Geometry: final body of the model. Coordinates: model frame, mm. Coordinates: 2 decimals unless noted, no trailing zeros. Order: outer loops, then holes, each group sorted by start corner. A loop starts at its lowest first (then second) coordinate and runs counter-clockwise, first axis right, second up. Notation, with made-up numbers: M 38.5,-34.5 L 46.5,-34.5 A24 ccw 46.5,-14.5 Z; hole C -19.75,-20.75 d7. An arc over 180 degrees is marked long. Use CSV: the item, a comma, the result in double quotes. Start each with the question number.
1. Section query B-B on z = 0.8. Return the cut outline in (x, y), and give its area (3 significant figures).
2. Section query D-D on x = -1200. Return the cut outline in (y, z), and give its area (3 significant figures).
3. Material intervals for line 1 (X direction, y = -220.5, z = 4.2); line 2 (Y direction, x = -1216.6, z = 3); line 3 (X direction, y = -244.5, z = 2.9), sorted ascending.
4. Section query C-C on x = -1019. Return the cut outline in (y, z), and give its area (3 significant figures).
5. Section query A-A on y = -232.5. Return the cut outline in (x, z), and give its area (4 significant figures).
6. First-contact query: P1, Ø4.5, axis at x = -957.6, y = -244.5, coming from the -Z side; P2, Ø1.5, axis at x = -1160, z = 1.5, coming from the +Y side. Flat tips, straight axial feed; report the tip coordinate or a pass-through.
from build123d import *

# Parameters (mm, degrees)
SKETCH1_W           = 267
SKETCH1_H           = 267.4
SKETCH1_R           = 2.5
SKETCH1_W_2         = 33
SKETCH1_H_2         = 90
BOSS_EXTRUDE1_DEPTH = 5
SKETCH6_W           = 267
SKETCH6_H           = 70.024397165
CUT_EXTRUDE4_DEPTH  = 6


with BuildPart() as part:
    # Sketch1 → Boss-Extrude1 (new body)
    with BuildSketch(Plane.XY):
        with Locations((-1087.1, -202.7)):
            Rectangle(SKETCH1_W, SKETCH1_H)
        with Locations((-957.6, -193.5)):
            Circle(SKETCH1_R, mode=Mode.SUBTRACT)
        with Locations((-957.6, -244.5)):
            Circle(SKETCH1_R, mode=Mode.SUBTRACT)
        with Locations((-1216.6, -244.5)):
            Circle(SKETCH1_R, mode=Mode.SUBTRACT)
        with Locations((-1216.6, -193.5)):
            Circle(SKETCH1_R, mode=Mode.SUBTRACT)
        with Locations((-1010.24, -219)):
            Rectangle(SKETCH1_W_2, SKETCH1_H_2, mode=Mode.SUBTRACT)
        with Locations((-1163.96, -219)):
            Rectangle(SKETCH1_W_2, SKETCH1_H_2, mode=Mode.SUBTRACT)
    extrude(amount=BOSS_EXTRUDE1_DEPTH)

    # Sketch6 → Cut-Extrude4 (cut, through all)
    with BuildSketch(Plane.XY.offset(5)):
        with BuildLine():
            Line((-1058.659911457, -69), (-953.6, -69))
            Line((-953.6, -69), (-953.6, -182))
            Line((-953.6, -182), (-980.204338358, -182))
            Line((-980.204338358, -182), (-980.204338358, -154))
            Line((-980.204338358, -154), (-1000.350392508, -154))
            ThreePointArc((-1000.350392508, -154), (-1051.889212828, -126.855339059), (-1058.659911457, -69))
        make_face()
        with Locations((-1087.1, -301.387801417)):
            Rectangle(SKETCH6_W, SKETCH6_H)
        with BuildLine():
            Line((-1115.540088543, -69), (-1220.6, -69))
            Line((-1220.6, -69), (-1220.6, -182))
            Line((-1220.6, -182), (-1193.995661642, -182))
            Line((-1193.995661642, -182), (-1193.995661642, -154))
            Line((-1193.995661642, -154), (-1173.849607492, -154))
            ThreePointArc((-1173.849607492, -154), (-1122.310787172, -126.855339059), (-1115.540088543, -69))
        make_face()
    extrude(amount=-CUT_EXTRUDE4_DEPTH, mode=Mode.SUBTRACT)


solid = part.part
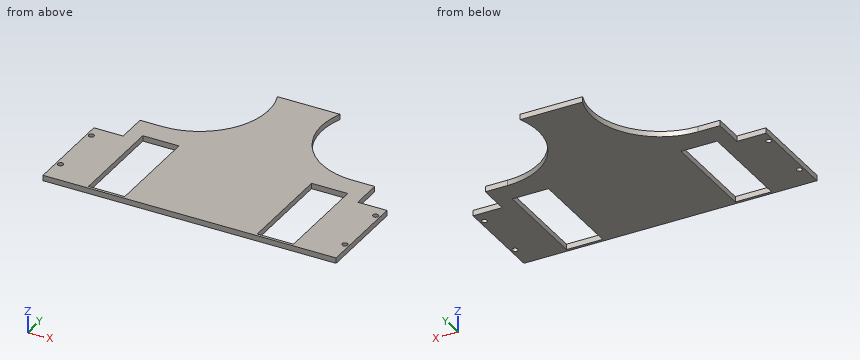
Results list:
1,outline,"M -1220.6,-266.38 L -953.6,-266.38 L -953.6,-182 L -980.2,-182 L -980.2,-154 L -1000.35,-154 A62.5 cw -1058.66,-69 L -1115.54,-69 A62.5 cw -1173.85,-154 L -1194,-154 L -1194,-182 L -1220.6,-182 Z; hole C -1216.6,-244.5 d5; hole C -1216.6,-193.5 d5; hole M -1180.46,-264 L -1147.46,-264 L -1147.46,-174 L -1180.46,-174 Z; hole M -1026.74,-264 L -993.74,-264 L -993.74,-174 L -1026.74,-174 Z; hole C -957.6,-244.5 d5; hole C -957.6,-193.5 d5"
1,area,"28,400 mm²"
2,outline,"M -266.38,0 L -182,0 L -182,5 L -266.38,5 Z"
2,area,"422 mm²"
3,line 1,"x = -1220.6 to -1180.46, -1147.46 to -1026.74, -993.74 to -953.6"
3,line 2,"y = -266.38 to -247, -242 to -196, -191 to -182"
3,line 3,"x = -1220.6 to -1219.1, -1214.1 to -1180.46, -1147.46 to -1026.74, -993.74 to -960.1, -955.1 to -953.6"
4,outline,"M -266.38,0 L -264,0 L -264,5 L -266.38,5 Z; M -174,0 L -151.15,0 L -151.15,5 L -174,5 Z"
4,area,"126 mm²"
5,outline,"M -1220.6,0 L -1180.46,0 L -1180.46,5 L -1220.6,5 Z; M -1147.46,0 L -1026.74,0 L -1026.74,5 L -1147.46,5 Z; M -993.74,0 L -953.6,0 L -953.6,5 L -993.74,5 Z"
5,area,"1,005 mm²"
6,P1,"passes through"
6,P2,"stops at y = -152.27"
